Here's the drawing with two shaded views (mm, measured from the low corner). I have some questions. A direction names the side the tool comes from. Round coordinates to 2 decimals unless told otherwise and drop trailing zeros. Loops run counter-clockwise (first coordinate to the right, second up) from the corner with the lowest first, then second, coordinate; pieces in that order, holes last.
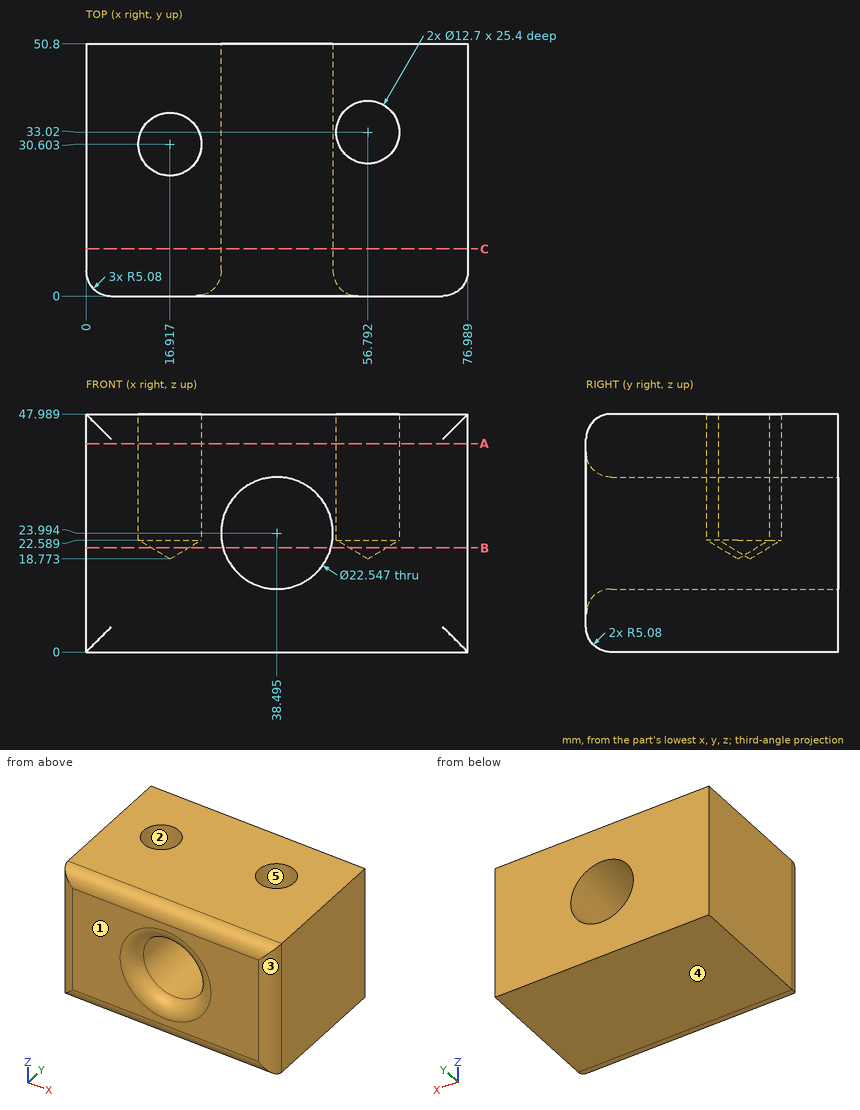
(1) If I drill on line 1 (X direction, y = 33, z = 34) (1 decimal); line 2 (Y direction, x = 14, z = 23) (1 decimal); line 3 (X direction, y = 10.5, z = 15), over which ranges is the centre line in solid material (lowest first)?
Worked answers:
line 1: x = 0 to 11, 22.8 to 33.3, 43.7 to 50.4, 63.1 to 77
line 2: y = 0 to 25, 36.2 to 50.8
line 3: x = 0 to 31.7, 45.29 to 76.99
(2) If we mould it in two halves opening along X, with no side actions, what happens to the marked faces 1, 2 and 3? For each: released by +X, released by -X, zero draft, split by the parting line, or undercut.
Worked answers:
face 1: zero draft
face 2: undercut
face 3: released by +X
(3) If we section it at C-C, the plane y = 9.5: List the corners of the cut face in (x, z) for me (1 decimal), then the cut area to 3 significant figures.
Worked answers:
outline: (0, 0) - (77, 0) - (77, 48) - (0, 48) - close; hole circle Ø22.5 at (38.5, 24)
area: 3,300 mm2
(4) For the marked faces 4 and 5, which set-ups out of +Z, -Z, +X, -X, +Y, -Y let a thin tool reach every point of the face, with its end or its side?
Worked answers:
face 4: -Z, +X, -X, +Y, -Y
face 5: +Z
(5) If we section it at B-B, the plane z = 21: State how many separate pieces and enclosed holes the cut face has, then the cut area to 3 significant figures.
Worked answers:
separate pieces: 2
enclosed holes: 2
area: 2,700 mm2
(6) If we section it at A-A, the plane z = 42: List the corners of the cut face in (x, y) for me.
Worked answers:
outline: (0, 5.08) arc R5.08 ccw to (5.08, 0) - (71.91, 0) arc R5.08 ccw to (76.99, 5.08) - (76.99, 50.8) - (0, 50.8) - close; hole circle Ø12.7 at (16.92, 30.6); hole circle Ø12.7 at (56.79, 33.02)
